Input: part model. Units: mm. Frame: model coordinates. A direction names the side the tool comes from. Give positions to 0.01 mm unless a question says otherwise; leave off trailing zeros. Loops run counter-clockwise (first coordinate to the right, second up) from the corner with the lowest first, then second, coordinate; pieces in that order, holes last. Notation, with made-up numbers: (-24, 80.25) - (-3, 80.25) arc R26 ccw to (-3, 95.25) - close; hole circle Ø5 at (-6, 6). An arc over 180 degrees is marked (long way). One line per item, written item: value.
Autodesk Fusion 360 part; units mm, degrees
sketch "Sketch2" plane through (0, 0, 0) normal (0, 1, 0) x (1, 0, 0)
  line L0 (0, 0) -> (64.5, 0)
  line L1 (64.5, 0) -> (64.5, -35.5)
  line L2 (64.5, -35.5) -> (0, -35.5)
  line L3 (0, -35.5) -> (0, 0)
  dimension "d5" = 64.5
  dimension "d6" = 35.5
extrude "Extrude2" add sketch "Sketch2" along normal blind 100 makes body 1
sketch "Sketch3" plane through (0, 0, 0) normal (-1, 0, 0) x (0, 0, 1)
  line L0 (0, 0) -> (35.5, 0)
  line L1 (35.5, 0) -> (35.5, 100)
  line L2 (35.5, 100) -> (0, 100)
  line L3 (0, 100) -> (0, 0)
  line L4 (0, 100) -> (64.5, 100)
  line L5 (64.5, 100) -> (64.5, 0)
  line L6 (64.5, 0) -> (0, 0)
  line L7 (0, 0) -> (0, 100)
  dimension "d9" = 64.5
  dimension "d10" = 100
extrude "Extrude3" add sketch "Sketch3" along normal blind 31.4 separate body contours L1 L4 L5 L6 makes body 2
extrude "Extrude4" add 1 faces at (0, 66.6667, 23.6667) along direction (-1, 0, 0) blind 31.4 on bodies 1 bodies 1 2
sketch "Sketch4" plane through (0, 0, 64.5) normal (0, 0, 1) x (1, 0, 0)
  line L0 (0, 0) -> (0, 100)
  line L1 (0, 100) -> (-31.4, 100)
  line L2 (-31.4, 100) -> (-31.4, 0)
  line L3 (-31.4, 0) -> (0, 0)
  line L4 (-31.4, 100) -> (33.1, 100)
  line L5 (33.1, 100) -> (33.1, 0)
  line L6 (33.1, 0) -> (-31.4, 0)
  line L7 (-31.4, 0) -> (-31.4, 100)
  dimension "d15" = 64.5
  dimension "d16" = 100
extrude "Extrude5" add sketch "Sketch4" along normal blind 31.4 bodies 1
sketch "Sketch5" plane through (33.1, 0, 0) normal (1, 0, 0) x (0, 0, -1)
  line L0 (-64.5, 0) -> (-64.5, 100)
  line L1 (-64.5, 100) -> (-95.9, 100)
  line L2 (-95.9, 100) -> (-95.9, 0)
  line L3 (-95.9, 0) -> (-64.5, 0)
  line L4 (-95.9, 100) -> (-31.4, 100)
  line L5 (-31.4, 100) -> (-31.4, 0)
  line L6 (-31.4, 0) -> (-95.9, 0)
  line L7 (-95.9, 0) -> (-95.9, 100)
  dimension "d19" = 64.5
  dimension "d20" = 100
extrude "Extrude6" add sketch "Sketch5" along normal blind 31.4 bodies 1
Item 1: Section A-A, the plane x = 8. Output: boundary loops of the cut face in (y, z).
Verdict:
outline: (0, 0) - (100, 0) - (100, 35.5) - (0, 35.5) - close; (0, 64.5) - (100, 64.5) - (100, 95.9) - (0, 95.9) - close
Item 2: Draft query along Z for faces 3 (the face through (16, 51, 64.5)), 4 (the face through (16, 51, 95.9)), 5 (the face through (16, 0, 26)). Return one class per face: pulls with the +Z half, pulls with the -Z half, needs draft (parallel to the pull), parting line crosses it, or undercut.
Verdict:
face 3: undercut
face 4: pulls with the +Z half
face 5: needs draft
Item 3: Section B-B, the plane y = 6.5. Output: boundary loops of the cut face in (x, z), and give its area (3 significant figures).
Verdict:
outline: (-31.4, 0) - (64.5, 0) - (64.5, 95.9) - (-31.4, 95.9) - close; hole (0, 35.5) - (33.1, 35.5) - (33.1, 64.5) - (0, 64.5) - close
area: 8,240 mm^2
Item 4: Access query for faces 1 (the face through (0, 51, 50)), 2 (the face through (64.5, 49, 47)). Directions: +Z, -Z, +X, -X, +Y, -Y. A direction counts if a zero-diameter tool reaches every point of the face in a straight line with its end or side. Return the directions, or none.
Verdict:
face 1: +Y, -Y
face 2: +Z, -Z, +X, +Y, -Y
Item 5: Material intervals for L1, parallel to X at y = 5, z = 43; L2, parallel to Z at x = 24.5, y = 20, sorted ascending.
Verdict:
L1: x = -31.4 to 0, 33.1 to 64.5
L2: z = 0 to 35.5, 64.5 to 95.9
Item 6: Pin query (flat end, axial travel): P1, Ø3, axis at x = 30.5, z = 34.5, coming from the -Y side. Return the tip coordinate at first contact, or that it passes through.
Verdict:
P1: stops at y = 0
